Geometry check sheet. Reference: drawing and pictorial views, mm from the part's lowest x, y, z. A direction names the side the tool comes from. Coordinates: 2 decimals unless noted, no trailing zeros. Loops run counter-clockwise (first coordinate to the right, second up) from the corner with the lowest first, then second, coordinate; pieces in that order, holes last. Notation, with made-up numbers: (56, -12) -> (70, -12) arc R25 cw to (70, 13) -> close; hole circle Ø6 at (-14.5, 38.5). An arc over 180 degrees is marked (long way). Answer as a JSON object with one key per item and string values. Group by question number.
Q1. Cross-section at D-D on x = 5.5. Record the boundary of the cut face in (y, z), and give its area (3 significant figures).
Q2. Cross-section at B-B on x = 14.5. Record the boundary of the cut face in (y, z) (1 decimal), and give its area (3 significant figures).
Q3. Cross-section at A-A on z = 40. Record the boundary of the cut face in (x, y), and give its area (4 significant figures).
Q4. Release check for a two-part mould opening along Y. For the marked faces 3, 4 and 5 record: released by +Y, released by -Y, zero draft, split by the parting line, or undercut.
Q5. Gauge pin test, flat ends, axial feed: pin 1 Ø1 at (x, y) = (13, 55.5) entering from -Z; pin 2 Ø1.5 at (x, z) = (31, 8) entering from -Y; pin 3 Ø4 at (x, y) = (5.5, 53) entering from -Z; pin 4 Ø2.5 at (y, z) = (40, 40) entering from +X. Record the tip position at first contact, or that the pin passes through.
Q6. Cross-section at C-C on z = 48.5. Record the boundary of the cut face in (x, y).
Q7. Set-up check for the marked faces 1 and 2: record each of +Z, -Z, +X, -X, +Y, -Y from which the full face is reachable in a straight line by a thin tool's end or side.
Q8. Scan lines: L1, parallel to Y at x = 4, z = 40; L2, parallel to X at y = 29, z = 36; L3, parallel to Z at x = 32, y = 54 (1 decimal). Record each from-to range of solid material in increasing order.
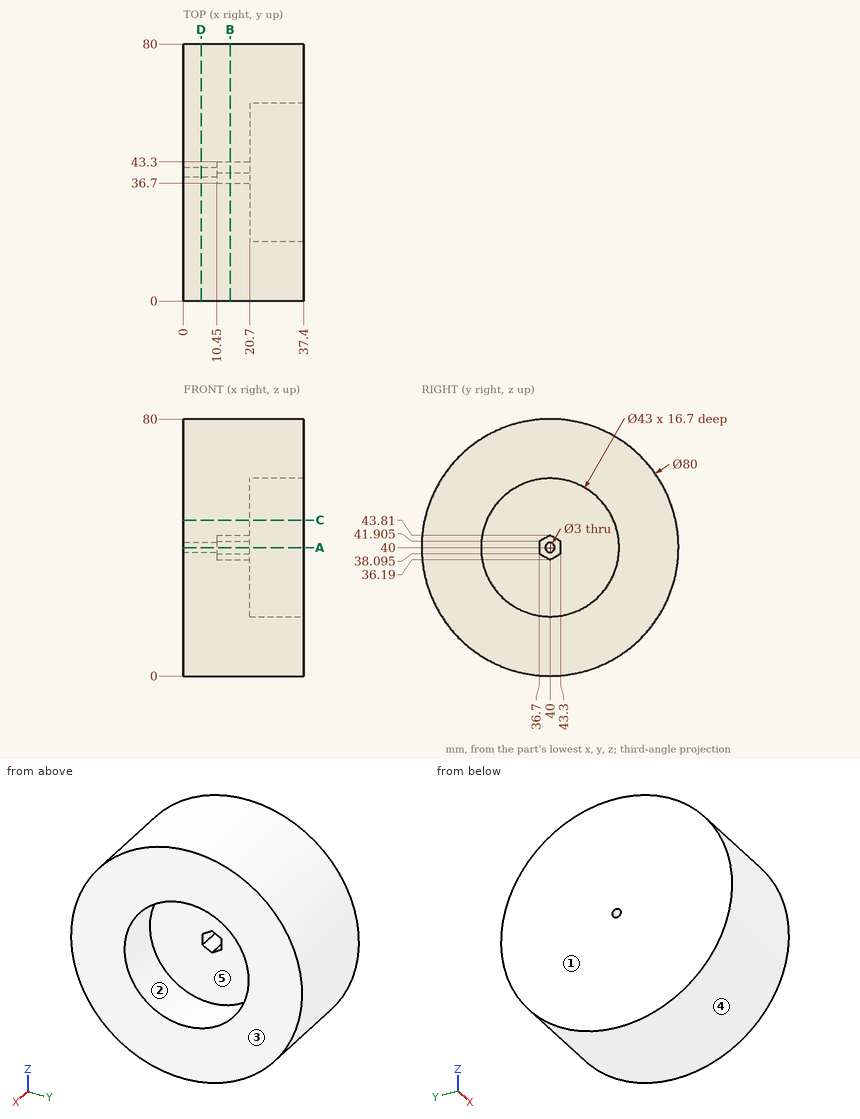
Computed values:
{
 "1": {"outline": "circle Ø80 at (40, 40); hole circle Ø3 at (40, 40)", "area": "5,020 mm²"},
 "2": {"outline": "circle Ø80 at (40, 40); hole (36.7, 38.1) -> (40, 36.2) -> (43.3, 38.1) -> (43.3, 41.9) -> (40, 43.8) -> (36.7, 41.9) -> close", "area": "4,990 mm²"},
 "3": {"outline": "(0, 0) -> (37.4, 0) -> (37.4, 18.5) -> (20.7, 18.5) -> (20.7, 36.7) -> (10.45, 36.7) -> (10.45, 38.5) -> (0, 38.5) -> close; (0, 41.5) -> (10.45, 41.5) -> (10.45, 43.3) -> (20.7, 43.3) -> (20.7, 61.5) -> (37.4, 61.5) -> (37.4, 80) -> (0, 80) -> close", "area": "2,175 mm²"},
 "4": {"face 3": "zero draft", "face 4": "split by the parting line", "face 5": "undercut"},
 "5": {"pin 1": "stops at z = 2.92", "pin 2": "stops at y = 15.03", "pin 3": "stops at z = 1.54", "pin 4": "passes through"},
 "6": {"outline": "(0, 0.91) -> (37.4, 0.91) -> (37.4, 20.25) -> (20.7, 20.25) -> (20.7, 59.75) -> (37.4, 59.75) -> (37.4, 79.09) -> (0, 79.09) -> close"},
 "7": {"face 1": "+Z, -Z, -X, +Y, -Y", "face 2": "+X"},
 "8": {"L1": "y = 0 to 38.5, 41.5 to 80", "L2": "x = 0 to 20.7", "L3": "z = 2.5 to 23.7, 56.3 to 77.5"}
}
